Can you work these out from the model? Positions are in its coordinate system, mm. A direction names the side the tool comes from. Coordinates: 2 decimals unless noted, no trailing zeros. Loops run counter-clockwise (first coordinate to the right, second up) from the corner with the lowest first, then second, coordinate; pieces in that order, holes last.
```python
from build123d import *

# Parameters (mm, degrees)
F0_R     = 7.0485
F1_DEPTH = 4.7498
F2_R     = 4.7625
F3_DEPTH = 0.254
F4_R     = 4.7625
F5_DEPTH = 0.254
F6_R     = 3.175
F7_DEPTH = 5.2588


with BuildPart() as f1:
    # F0 (on Top) → F1 (new body)
    with BuildSketch(Plane.XY):
        Circle(F0_R)
    extrude(amount=F1_DEPTH)

    # F2 (on face) → F3 (join)
    with BuildSketch(Plane(origin=(0, 0, 0), x_dir=(1, 0, 0), z_dir=(0, 0, -1))):
        Circle(F2_R)
    extrude(amount=F3_DEPTH)

    # F4 (on face) → F5 (join)
    with BuildSketch(Plane.XY.offset(4.7498)):
        Circle(F4_R)
    extrude(amount=F5_DEPTH)

    # F6 (on face) → F7 (cut, through all)
    with BuildSketch(Plane(origin=(0, 0, -0.254), x_dir=(1, 0, 0), z_dir=(0, 0, -1))):
        Circle(F6_R)
    extrude(amount=-F7_DEPTH, mode=Mode.SUBTRACT)


solid = f1.part
```
Item 1: I'm going to push flat-ended pins straight in: P1, Ø1.5, axis at x = 5.5, z = 2, coming from the -Y side; P2, Ø1.5, axis at x = -5.5, y = 1, coming from the +Z side; P3, Ø1.5, axis at x = 5.5, z = 1.5, coming from the +Y side; P4, Ø5.5, axis at x = 0, y = 0, coming from the +Z side. Where does each tip first touch, or does it pass through?
Results are:
P1: stops at y = -5.21
P2: stops at z = 4.75
P3: stops at y = 5.21
P4: passes through
Item 2: On a 3-axis mill with a long thin cutter (end or side, diameter ignored), from which of +Z, -Z, +X, -X, +Y, -Y can I reach the whole of each face in a straight line? I mean faces 1 (the face through (1, -5, 0)), 2 (the face through (-0.69, 3.1, 2.34)), 3 (the face through (1, -5, 4.75)). Say none if no direction works.
Results are:
face 1: -Z
face 2: +Z, -Z
face 3: +Z
Item 3: Suppose I cut it at D-D, the plane y = 4. Please give me the cut outline in (x, z), plus the area to 3 significant figures.
Results are:
outline: (-5.8, 0) - (-2.58, 0) - (-2.58, -0.25) - (2.58, -0.25) - (2.58, 0) - (5.8, 0) - (5.8, 4.75) - (2.58, 4.75) - (2.58, 5) - (-2.58, 5) - (-2.58, 4.75) - (-5.8, 4.75) - close
area: 57.8 mm2
Item 4: I need wall thicknesses on line 1 along Y through (x, z) = (0, 3.45) (1 decimal); line 2 along X through (y, z) = (0.5, 3.95); line 3 along Y through (x, z) = (-1.25, 2.25). Which ranges of each line are inside material? Lowest first, please.
Results are:
line 1: y = -7 to -3.2, 3.2 to 7
line 2: x = -7.03 to -3.14, 3.14 to 7.03
line 3: y = -6.94 to -2.92, 2.92 to 6.94
